from build123d import *

# Parameters (mm, degrees)
SKETCH_1_R          = 28.5
EXTRUDE_1_DEPTH     = 52.25
SKETCH_3_R          = 17.5
CUT_EXTRUDE_2_DEPTH = 10
SKETCH_4_R          = 1.7
CUT_EXTRUDE_3_DEPTH = 10
SKETCH_5_R          = 1.5
CUT_EXTRUDE_4_DEPTH = 10


with BuildPart() as part:
    # 草图1 → 凸台-拉伸1 (new body)
    with BuildSketch(Plane(origin=(0, 0, 0), x_dir=(1, 0, 0), z_dir=(0, 1, 0))):
        Circle(SKETCH_1_R)
    extrude(amount=EXTRUDE_1_DEPTH)

    # 草图3 → 切除-拉伸2 (cut)
    with BuildSketch(Plane(origin=(0, 52.25, 0), x_dir=(1, 0, 0), z_dir=(0, 1, 0))):
        Circle(SKETCH_3_R)
    extrude(amount=-CUT_EXTRUDE_2_DEPTH, mode=Mode.SUBTRACT)

    # 草图4 → 切除-拉伸3 (cut)
    with BuildSketch(Plane(origin=(0, 52.25, 0), x_dir=(1, 0, 0), z_dir=(0, 1, 0))):
        with Locations((17.67766953, -17.67766953)):
            Circle(SKETCH_4_R)
        with Locations((-6.470476128, -24.148145657)):
            Circle(SKETCH_4_R)
        with Locations((-24.148145657, -6.470476128)):
            Circle(SKETCH_4_R)
        with Locations((-17.67766953, 17.67766953)):
            Circle(SKETCH_4_R)
        with Locations((6.470476128, 24.148145657)):
            Circle(SKETCH_4_R)
        with Locations((24.148145657, 6.470476128)):
            Circle(SKETCH_4_R)
    extrude(amount=-CUT_EXTRUDE_3_DEPTH, mode=Mode.SUBTRACT)

    # 草图5 → 切除-拉伸4 (cut)
    with BuildSketch(Plane.XZ):
        with Locations((0, -19)):
            Circle(SKETCH_5_R)
        with Locations((-19, 0)):
            Circle(SKETCH_5_R)
        with Locations((0, 19)):
            Circle(SKETCH_5_R)
        with Locations((19, 0)):
            Circle(SKETCH_5_R)
    extrude(amount=-CUT_EXTRUDE_4_DEPTH, mode=Mode.SUBTRACT)


solid = part.part
Could you check a few things on this model? Use its own coordinates, in mm. A direction names the side the tool comes from. Give positions to 0.01 mm unless a question says otherwise; leave off trailing zeros. Order: outer loops, then holes, each group sorted by start corner. A loop starts at its lowest first (then second) coordinate and runs counter-clockwise, first axis right, second up.
1. Suppose I cut it at B-B (y = 44). Write out the boundary of the cut face in (x, z), plus the area to 3 significant figures.
Answers below:
outline: circle Ø57 at (0, 0); hole circle Ø3.4 at (-24.15, 6.47); hole circle Ø3.4 at (-17.68, -17.68); hole circle Ø35 at (0, 0); hole circle Ø3.4 at (-6.47, 24.15); hole circle Ø3.4 at (6.47, -24.15); hole circle Ø3.4 at (17.68, 17.68); hole circle Ø3.4 at (24.15, -6.47)
area: 1,540 mm2
2. Suppose I cut it at A-A (z = 0). Write out the boundary of the cut face in (x, y).
Answers below:
outline: (-28.5, 0) - (-20.5, 0) - (-20.5, 10) - (-17.5, 10) - (-17.5, 0) - (17.5, 0) - (17.5, 10) - (20.5, 10) - (20.5, 0) - (28.5, 0) - (28.5, 52.25) - (17.5, 52.25) - (17.5, 42.25) - (-17.5, 42.25) - (-17.5, 52.25) - (-28.5, 52.25) - close
3. For pin 1 (1.5 mm diameter, centred on y = 34.5, z = 4, fed in from -X); pin 2 (2.5 mm diameter, centred on x = 6.47, z = -24.15, fed in from +Y); pin 3 (1 mm diameter, centred on y = 26, z = -20.5, fed in from +X), each with a flat end and sliding along its axis, tell me the tip position at first contact or that it passes through.
Answers below:
pin 1: stops at x = -28.31
pin 2: stops at y = 42.25
pin 3: stops at x = 20.3
4. Suppose I cut it at C-C (y = 8.5). Write out the boundary of the cut face in (x, z).
Answers below:
outline: circle Ø57 at (0, 0); hole circle Ø3 at (-19, 0); hole circle Ø3 at (0, -19); hole circle Ø3 at (0, 19); hole circle Ø3 at (19, 0)
5. I need wall thicknesses on L1, parallel to Z at x = 0, y = 7.25; L2, parallel to Z at x = 0, y = 47.5; L3, parallel to X at y = 44, z = -6. Which ranges of each line are inside material? Lowest first, please.
Answers below:
L1: z = -28.5 to -20.5, -17.5 to 17.5, 20.5 to 28.5
L2: z = -28.5 to -17.5, 17.5 to 28.5
L3: x = -27.86 to -16.44, 16.44 to 22.51, 25.78 to 27.86
6. Which directions (+Z, -Z, +X, -X, +Y, -Y) give clear straight access to the entire face, cutting with the end or side of a thin tool? Please do faces 1 (the flat face through (0, 0, 0)), 2 (the flat face through (19, 10, 0)), 3 (the flat face through (0, 42.25, 0)).
Answers below:
face 1: +Z, -Z, +X, -X, -Y
face 2: -Y
face 3: +Y
7. Suppose I cut it at D-D (x = 0.5). Write out the boundary of the cut face in (y, z), plus the area to 3 significant figures.
Answers below:
outline: (0, -28.5) - (52.25, -28.5) - (52.25, -17.49) - (42.25, -17.49) - (42.25, 17.49) - (52.25, 17.49) - (52.25, 28.5) - (0, 28.5) - (0, 20.41) - (10, 20.41) - (10, 17.59) - (0, 17.59) - (0, -17.59) - (10, -17.59) - (10, -20.41) - (0, -20.41) - close
area: 2,570 mm2
8. Thinking about a two-plate mould opening in X: for faces 4 (the cylindrical face through (-0.195, 4.93, 20.487)), 5 (the cylindrical face through (26.327, 25.759, 10.916)), 6 (the flat face through (-13, 52.25, 12)), which applies, +X half, -X half, draft (parallel to the pull), parting line (faces both ways), or undercut?
Answers below:
face 4: undercut
face 5: parting line
face 6: draft
